Autodesk Inventor part; units mm, degrees
ref_plane "YZ Plane" through (0, 0, 0) normal (1, 0, 0) x (0, 1, 0)
ref_plane "XZ Plane" through (0, 0, 0) normal (0, 1, 0) x (-1, 0, 0)
ref_plane "XY Plane" through (0, 0, 0) normal (0, 0, 1) x (1, 0, 0)
sketch "Эскиз1" plane through (0, 0, 0) normal (0, 0, 1) x (1, 0, 0)
  line L0 (-40, 23) -> (40, 23)
  line L1 (40, 23) -> (40, -23)
  line L2 (40, -23) -> (-40, -23)
  line L3 (-40, -23) -> (-40, 23)
  line L4 (-40, 23) -> (40, -23) construction
  line L5 (40, 23) -> (-40, -23) construction
  point P0 (0, 0)
  dimension "d0" = 80
  dimension "d1" = 46
extrude "Выдавливание1" add sketch "Эскиз1" along normal blind 4
sketch "Эскиз2" plane through (-40, 23, 0) normal (0, 1, 0) x (1, 0, 0)
  line L0 (0, -4) -> (80, -4)
  line L1 (0, 0) -> (80, 0)
  line L2 (0, -4) -> (20, -4)
  line L3 (20, -4) -> (20, 0)
  line L4 (20, 0) -> (0, 0)
  line L5 (0, 0) -> (0, -4)
  line L6 (80, -4) -> (60, -4)
  line L7 (60, -4) -> (60, 0)
  line L8 (60, 0) -> (80, 0)
  line L9 (80, 0) -> (80, -4)
  line L10 (50, -4) -> (30, -4)
  line L11 (30, -4) -> (30, 0)
  line L12 (30, 0) -> (50, 0)
  line L13 (50, 0) -> (50, -4)
  point P0 (40, 0)
  point P1 (30, -2)
  point P2 (20, -2)
  point P3 (60, -2)
  point P4 (50, -2)
  dimension "d4" = 10
  dimension "d6" = 20
extrude "Выдавливание2" add sketch "Эскиз2" along normal blind 4 contours L5 L1 L3 L0 | L11 L1 L13 L0 | L7 L1 L9 L0
properties part number "стенка"
Verification items for the finished model (mm, model axes). A direction names the side the tool comes from. Give positions to 0.01 mm unless a question says otherwise; leave off trailing zeros. Loops run counter-clockwise (first coordinate to the right, second up) from the corner with the lowest first, then second, coordinate; pieces in that order, holes last. Notation, with made-up numbers: M -20,-19.5 L -15,-19.5 A28 cw -15,5.5 Z; hole C 46.5,65.5 d5. An arc over 180 degrees is marked long. Return JSON: item names as keys, results as strings.
1) Gauge pin test, flat end, axial feed: P1, Ø2, axis at x = 16, z = 1, coming from the +Y side. Record the tip position at first contact, or that the pin passes through.
Findings:
{"P1": "stops at y = 23"}
2) Section check B-B, the plane x = 13.5. Enter the section's corners in (y, z).
Findings:
{"outline": "M -23,0 L 23,0 L 23,4 L -23,4 Z"}
3) Material ranges on L1, parallel to Y at x = -10.5, z = 0.75, recorded low to high. Write a range as [from, to].
Findings:
{"L1": "y = [-23, 23]"}
4) Tool access check on faces 1 (the flat face through (-15, 23, 2)), 2 (the flat face through (-30, 27, 2)). Record the directions out of +Z, -Z, +X, -X, +Y, -Y that give a thin tool (end or side, any length) a straight path to the whole face; none if there is none.
Findings:
{"face 1": "+Z, -Z, +Y", "face 2": "+Z, -Z, +X, -X, +Y"}
5) Mould release check, pull along X, two halves, no side actions. Record for faces 3 (the flat face through (20, 25, 2)), 4 (the flat face through (10, 25, 2)), 5 (the flat face through (-1, 2, 4)), 6 (the flat face through (40, 2, 2)): released by +X, released by -X, zero draft, split by the parting line, or undercut.
Findings:
{"face 3": "undercut", "face 4": "undercut", "face 5": "zero draft", "face 6": "released by +X"}
6) Section check A-A, the plane z = 1.25. Enter the section's corners in (x, y).
Findings:
{"outline": "M -40,-23 L 40,-23 L 40,27 L 20,27 L 20,23 L 10,23 L 10,27 L -10,27 L -10,23 L -20,23 L -20,27 L -40,27 Z"}
